The figure shows three views and two pictorial views of one solid part (mm, origin at its lowest corner). Answer the questions. A direction names the side the tool comes from. Coordinates: 2 decimals unless noted, no trailing zeros. Loops run counter-clockwise (first coordinate to the right, second up) from the corner with the lowest first, then second, coordinate; pieces in that order, holes last.
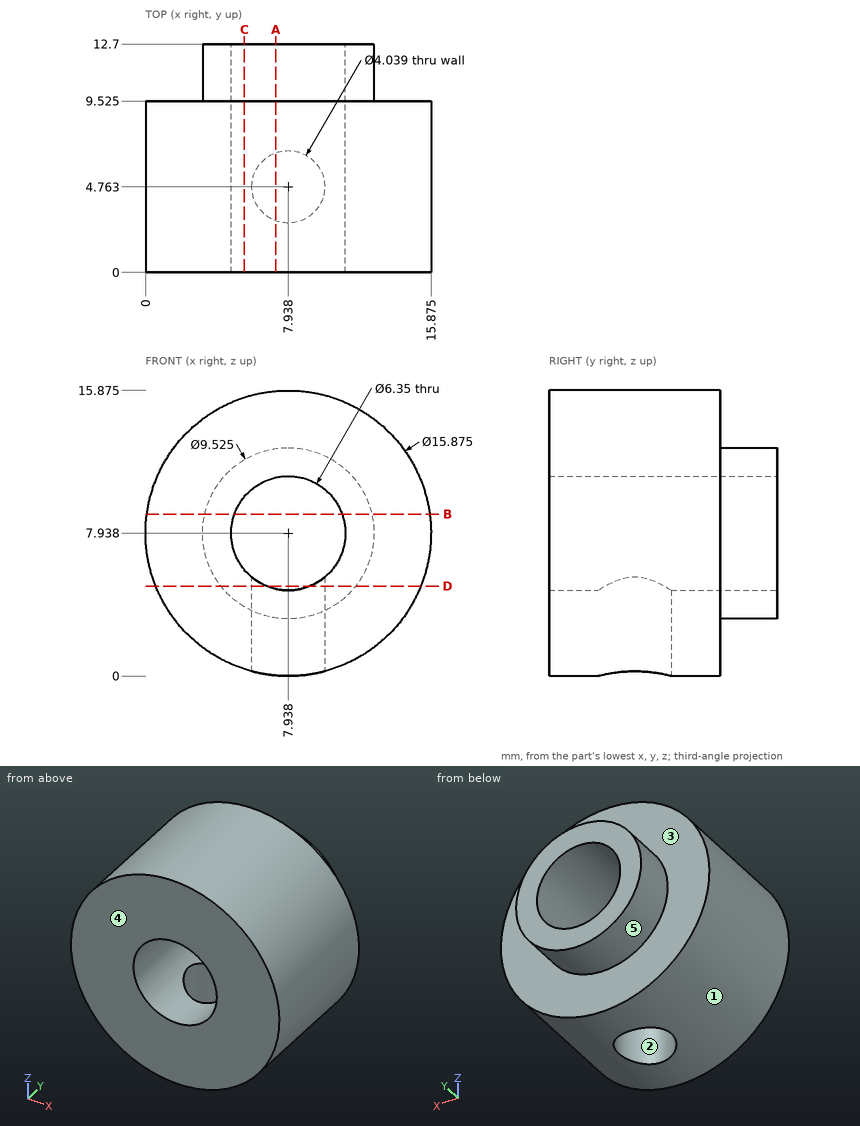
Q1. Determine the mould class of the marked faces 1, 2 and 3 for opening direction X: +X half, -X half, draft (parallel to the pull), parting line (faces both ways), or undercut.
Findings below:
face 1: parting line
face 2: undercut
face 3: draft
Q2. A cutting plane is placed at D-D (z = 5). Give the vertices of the cut face in (x, y) (1 decimal).
Findings below:
outline: (0.6, 0) - (6.7, 0) - (6.7, 3.1) arc R2 cw to (6.7, 6.4) - (6.7, 12.7) - (4.2, 12.7) - (4.2, 9.5) - (0.6, 9.5) - close; (9.1, 0) - (15.3, 0) - (15.3, 9.5) - (11.7, 9.5) - (11.7, 12.7) - (9.1, 12.7) - (9.1, 6.4) arc R2 cw to (9.1, 3.1) - close
Q3. A cutting plane is placed at C-C (x = 5.5). Give the vertices of the cut face in (y, z) (1 decimal), then the cut area to 3 significant figures.
Findings below:
outline: (0, 0.4) - (9.5, 0.4) - (9.5, 3.8) - (12.7, 3.8) - (12.7, 5.9) - (0, 5.9) - close; (0, 10) - (12.7, 10) - (12.7, 12) - (9.5, 12) - (9.5, 15.5) - (0, 15.5) - close
area: 118 mm2
Q4. A cutting plane is placed at A-A (x = 7.25). Count the separate pieces of the cut face and the enclosed holes in it.
Findings below:
separate pieces: 3
enclosed holes: 0
Q5. A cutting plane is placed at B-B (z = 9). Give the vertices of the cut face in (x, y) (1 decimal), then the cut area to 3 significant figures.
Findings below:
outline: (0.1, 0) - (4.9, 0) - (4.9, 12.7) - (3.3, 12.7) - (3.3, 9.5) - (0.1, 9.5) - close; (10.9, 0) - (15.8, 0) - (15.8, 9.5) - (12.6, 9.5) - (12.6, 12.7) - (10.9, 12.7) - close
area: 103 mm2
Q6. Straight lines are drawn through the part: probe 1 along Y at (x, z) = (14.75, 11.5) (1 decimal); probe 2 along X at (y, z) = (1, 9) (1 decimal); probe 3 along X at (y, z) = (12, 9) (1 decimal). For each, find the intervals that lie inside material, in ascending order.
Findings below:
probe 1: y = 0 to 9.5
probe 2: x = 0.1 to 4.9, 10.9 to 15.8
probe 3: x = 3.3 to 4.9, 10.9 to 12.6
Q7. Which of the six approach directions +Z, -Z, +X, -X, +Y, -Y give full straight-line access (tool end or side, diameter ignored) to the marked faces 4 and 5?
Findings below:
face 4: +Z, -Z, +X, -X, -Y
face 5: +Y
Q8. Flat-ended cylindrical pins translate along their axes: pin 1 Ø2 at (x, z) = (1.5, 13.5) entering from -Y; pin 2 Ø1.5 at (y, z) = (9.5, 2) entering from +X (1 decimal). Find the tip coordinate at first contact, or state that the pin passes through.
Findings below:
pin 1: stops at y = 0
pin 2: stops at x = 13.9
